Check sheet for the modelled part. Datum: model origin and axes. Units: mm. Face numbers are marked on the shaded views. A direction names the side the tool comes from. Give positions to 0.01 mm unless a question says otherwise; leave off trailing zeros. Loops run counter-clockwise (first coordinate to the right, second up) from the corner with the lowest first, then second, coordinate; pieces in that order, holes last. Notation, with made-up numbers: (-18, -39) - (1, -39) arc R26 cw to (1, -6) - close; hole circle Ø4 at (74.5, 11.25). An arc over 180 degrees is marked (long way). Answer in a Markdown table with one row per item. Add a question column.
(1) Sectioned sample at B-B on y = 0. Enter the section's corners in (x, z), then the cut area to 3 significant figures.
(2) Set-up check for the marked faces 5 and 6: record each of +Z, -Z, +X, -X, +Y, -Y from which the full face is reachable in a straight line by a thin tool's end or side.
(3) Sectioned sample at D-D on x = 0. Enter the section's corners in (y, z), then the cut area to 3 significant figures.
(4) Draft check along Y on the marked faces 1, 2, 3 and 4. Enter one of: released by +Y, released by -Y, zero draft, split by the parting line, or undercut.
(5) Sectioned sample at A-A on x = 15. Enter the section's corners in (y, z).
(6) Thickness scan on L1, parallel to Y at x = -15, z = 2.75; L2, parallel to Z at x = -17.5, y = 11.25; L3, parallel to X at y = 4.75, z = 10.5. Record the ranges inside material, lowest first.
(7) Sectioned sample at C-C on z = 3.5. Enter the section's corners in (x, y).
(8) Go/stop test with flat-tipped pins: P1, Ø2.5, axis at x = -3.5, y = 7.5, coming from the +Z side; P2, Ø1.5, axis at x = -1, y = 7.5, coming from the +Z side; P3, Ø2, axis at y = -1.5, z = 15, coming from the -X side. Record where each tip stops, or that it passes through.
from build123d import *

# Parameters (mm, degrees)
SKETCH_W        = 50
SKETCH_H        = 25
SKETCH_R        = 3.1
PAD_DEPTH       = 4
SKETCH001_W     = 10
SKETCH001_H     = 25
PAD001_DEPTH    = 15
SKETCH002_R     = 2.1
POCKET_DEPTH    = 25.001
FILLET_R        = 3
SKETCH003_W     = 3
SKETCH003_H     = 3
POCKET001_DEPTH = 30.001
CHAMFER_SIZE    = 1
FILLET001_R     = 2


with BuildPart() as part:
    # Sketch → Pad (new body)
    with BuildSketch(Plane.XY):
        Rectangle(SKETCH_W, SKETCH_H)
        with Locations((-15, 0)):
            Circle(SKETCH_R, mode=Mode.SUBTRACT)
        with Locations((15, 0)):
            Circle(SKETCH_R, mode=Mode.SUBTRACT)
    extrude(amount=PAD_DEPTH)

    # Sketch001 (on Face8 of Pad) → Pad001 (join)
    with BuildSketch(Plane.XY.offset(4)):
        Rectangle(SKETCH001_W, SKETCH001_H)
    extrude(amount=PAD001_DEPTH)

    # Sketch002 (on Face14 of Pad001) → Pocket (cut, through all)
    with BuildSketch(Plane.XZ.offset(12.5)):
        with Locations((0, 17.669756)):
            Circle(SKETCH002_R)
    extrude(amount=-POCKET_DEPTH, mode=Mode.SUBTRACT)

    # Fillet
    fillet_edges = [part.edges().sort_by_distance(p)[0] for p in [
        (5, 0, 19),
        (-5, 0, 19),
    ]]
    fillet(fillet_edges, radius=FILLET_R)

    # Sketch003 (on Face2 of Fillet) → Pocket001 (cut, through all)
    with BuildSketch(Plane.YZ.offset(5)):
        with Locations((-7, 17.5)):
            Rectangle(SKETCH003_W, SKETCH003_H)
        with Locations((7, 17.5)):
            Rectangle(SKETCH003_W, SKETCH003_H)
        with Locations((-7, 9.5)):
            Rectangle(SKETCH003_W, SKETCH003_H)
        with Locations((7, 9.5)):
            Rectangle(SKETCH003_W, SKETCH003_H)
    extrude(amount=-POCKET001_DEPTH, mode=Mode.SUBTRACT)

    # Chamfer
    chamfer_edges = [part.edges().sort_by_distance(p)[0] for p in [
        (-25, -12.5, 2),
        (25, -12.5, 2),
        (25, 12.5, 2),
        (-25, 12.5, 2),
        (-15, 12.5, 4),
        (-25, 0, 4),
        (-15, -12.5, 4),
        (15, -12.5, 4),
        (25, 0, 4),
        (15, 12.5, 4),
    ]]
    chamfer(chamfer_edges, length=CHAMFER_SIZE)

    # Fillet001
    fillet001_edges = [part.edges().sort_by_distance(p)[0] for p in [
        (-5, 0, 4),
        (5, 0, 4),
    ]]
    fillet(fillet001_edges, radius=FILLET001_R)


solid = part.part
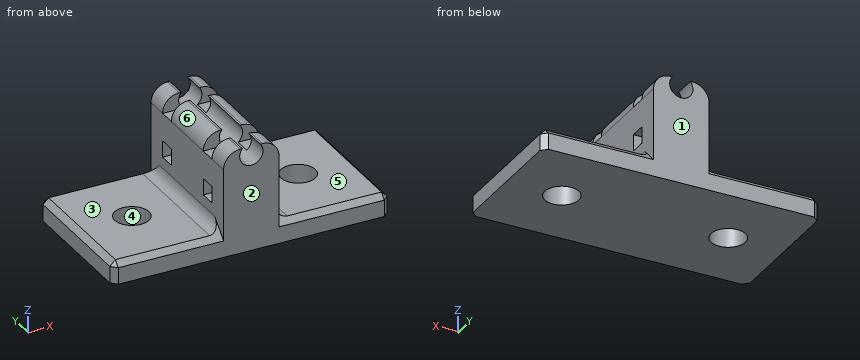
Reply:
| question | item | result |
|---|---|---|
| 1 | outline | (-25, 0) - (-18.1, 0) - (-18.1, 4) - (-24, 4) - (-25, 3) - close; (-11.9, 0) - (11.9, 0) - (11.9, 4) - (7, 4) arc R2 cw to (5, 6) - (5, 16) arc R3 ccw to (2, 19) - (1.62, 19) arc R2.1 cw (long way) to (-1.62, 19) - (-2, 19) arc R3 ccw to (-5, 16) - (-5, 6) arc R2 cw to (-7, 4) - (-11.9, 4) - close; (18.1, 0) - (25, 0) - (25, 3) - (24, 4) - (18.1, 4) - close |
| 1 | area | 285 mm^2 |
| 2 | face 5 | +Z, +X, +Y, -Y |
| 2 | face 6 | +Z, -X, +Y, -Y |
| 3 | outline | (-12.5, 0) - (12.5, 0) - (12.5, 15.57) - (-12.5, 15.57) - close; hole (-8.5, 8) - (-5.5, 8) - (-5.5, 11) - (-8.5, 11) - close; hole (5.5, 8) - (8.5, 8) - (8.5, 11) - (5.5, 11) - close |
| 3 | area | 371 mm^2 |
| 4 | face 1 | released by +Y |
| 4 | face 2 | released by -Y |
| 4 | face 3 | zero draft |
| 4 | face 4 | undercut |
| 5 | outline | (-12.5, 0) - (-3.1, 0) - (-3.1, 4) - (-11.5, 4) - (-12.5, 3) - close; (3.1, 0) - (12.5, 0) - (12.5, 3) - (11.5, 4) - (3.1, 4) - close |
| 6 | L1 | -12.5 to -3.1, 3.1 to 12.5 |
| 6 | L2 | 0 to 4 |
| 6 | L3 | -5 to 5 |
| 7 | outline | (-24.5, -11.5) - (-24, -12) - (-5, -12) - (-5, -12.5) - (5, -12.5) - (5, -12) - (24, -12) - (24.5, -11.5) - (24.5, 11.5) - (24, 12) - (5, 12) - (5, 12.5) - (-5, 12.5) - (-5, 12) - (-24, 12) - (-24.5, 11.5) - close; hole circle Ø6.2 at (-15, 0); hole circle Ø6.2 at (15, 0) |
| 8 | P1 | z = 18.9 |
| 8 | P2 | z = 16 |
| 8 | P3 | x = -5 |
